The listing builds one solid part. Answer for the finished solid, in the listing's coordinates (mm). A direction names the side the tool comes from. Round coordinates to 2 decimals unless told otherwise and drop trailing zeros. Loops run counter-clockwise (first coordinate to the right, second up) from the corner with the lowest first, then second, coordinate; pieces in that order, holes last. Notation, with made-up numbers: (-15, -29) -> (31, -29) arc R14 cw to (31, -2) -> close; hole circle Ø8 at (-9.5, -4.5). An arc over 180 degrees is marked (long way). Write each question's results on one line, items separated by ' | '. Start each with the question number.
(1) For faces 1 (the face through (299, -290.364, 49)), 2 (the face through (242.644, -285.339, 49.3)), determine the directions among +Z, -Z, +X, -X, +Y, -Y from which every point of the face is accessible in a straight line to the end or side of a thin tool.
(2) The part is cut by section B-B (y = -272.5). Determine the outline of the cut face in (x, z).
(3) The part is cut by section A-A (x = 254.5). Determine the outline of the cut face in (y, z), plus the area to 3 significant figures.
(4) Determine the mould class of faces 3 (the face through (357.494, -285.24, 49.3)), 4 (the face through (240.41, -287.63, 49.3)), 5 (the face through (301, -215.364, 49)), 6 (the face through (359.78, -287.48, 49.3)) for opening direction X: released by +X, released by -X, zero draft, split by the parting line, or undercut.
(5) Straight lines are drawn through the part: probe 1 along X at (y, z) = (-248, 60.5); probe 2 along Y at (x, z) = (347.5, 91.5); probe 3 along X at (y, z) = (-224, 74.5). For each, find the intervals that lie inside material, in ascending order.
(6) The part is cut by section C-C (z = 53.5). Determine the outline of the cut face in (x, y), plus the area to 3 significant figures.
Autodesk Fusion 360 part; units mm, degrees
sketch "スケッチ1" plane through (0, 0, 0) normal (0, 0, 1) x (1, 0, 0)
  line L0 (247.1191, -287.1642) -> (352.9191, -287.1642)
  line L1 (352.9191, -215.3642) -> (247.1191, -215.3642)
  line L2 (352.9191, -218.5642) -> (247.1191, -218.5642)
  line L3 (237.5191, -224.9642) -> (237.5191, -280.7642)
  line L4 (240.7191, -224.9642) -> (240.7191, -280.7642)
  arc A0 (240.7191, -280.7642) -> (247.1191, -287.1642) centre (247.1191, -280.7642) ccw
  arc A1 (247.1191, -215.3642) -> (237.5191, -224.9642) centre (247.1191, -224.9642) ccw
  arc A2 (247.1191, -218.5642) -> (240.7191, -224.9642) centre (247.1191, -224.9642) ccw
  line L5 (362.5191, -280.7642) -> (362.5191, -224.9642)
  line L6 (359.3191, -280.7642) -> (359.3191, -224.9642)
  arc A3 (352.9191, -287.1642) -> (359.3191, -280.7642) centre (352.9191, -280.7642) ccw
  arc A4 (362.5191, -224.9642) -> (352.9191, -215.3642) centre (352.9191, -224.9642) ccw
  arc A5 (359.3191, -224.9642) -> (352.9191, -218.5642) centre (352.9191, -224.9642) ccw
  line L7 (247.1191, -290.3642) -> (352.9191, -290.3642)
  arc A6 (237.5191, -280.7642) -> (247.1191, -290.3642) centre (247.1191, -280.7642) ccw
  arc A7 (352.9191, -290.3642) -> (362.5191, -280.7642) centre (352.9191, -280.7642) ccw
  point P0 (300.0191, -252.8642)
extrude "押し出し1" add sketch "スケッチ1" along normal blind 100
Checked values:
1) face 1: +Z, -Z, +X, -X, -Y | face 2: +Z, -Z
2) outline: (237.52, 0) -> (240.72, 0) -> (240.72, 100) -> (237.52, 100) -> close; (359.32, 0) -> (362.52, 0) -> (362.52, 100) -> (359.32, 100) -> close
3) outline: (-290.36, 0) -> (-287.16, 0) -> (-287.16, 100) -> (-290.36, 100) -> close; (-218.56, 0) -> (-215.36, 0) -> (-215.36, 100) -> (-218.56, 100) -> close | area: 640 mm2
4) face 3: undercut | face 4: released by -X | face 5: zero draft | face 6: released by +X
5) probe 1: x = 237.52 to 240.72, 359.32 to 362.52 | probe 2: y = -290.36 to -287.16, -218.56 to -215.36 | probe 3: x = 237.57 to 240.79, 359.25 to 362.47
6) outline: (237.52, -280.76) arc R9.6 ccw to (247.12, -290.36) -> (352.92, -290.36) arc R9.6 ccw to (362.52, -280.76) -> (362.52, -224.96) arc R9.6 ccw to (352.92, -215.36) -> (247.12, -215.36) arc R9.6 ccw to (237.52, -224.96) -> close; hole (240.72, -280.76) arc R6.4 ccw to (247.12, -287.16) -> (352.92, -287.16) arc R6.4 ccw to (359.32, -280.76) -> (359.32, -224.96) arc R6.4 ccw to (352.92, -218.56) -> (247.12, -218.56) arc R6.4 ccw to (240.72, -224.96) -> close | area: 1,200 mm2
